Autodesk Inventor part; units mm, degrees
ref_plane "YZ Plane" through (0, 0, 0) normal (1, 0, 0) x (0, 1, 0)
ref_plane "XZ Plane" through (0, 0, 0) normal (0, 1, 0) x (-1, 0, 0)
ref_plane "XY Plane" through (0, 0, 0) normal (0, 0, 1) x (1, 0, 0)
sketch "Sketch1" plane through (0, 0, 0) normal (0, 1, 0) x (-1, 0, 0)
  circle A0 centre (0, 0) radius 8.5
  line L0 (10, -11.1988) -> (10, 11.1988)
  line L1 (-10, 11.1988) -> (-10, -11.1988)
  line L2 (-10, -14.792) -> (10, 14.792) construction
  line L3 (10, -14.792) -> (-10, 14.792) construction
  line L4 (10, 11.1988) -> (-10, 11.1988) construction
  arc A1 (10, 11.1988) -> (-10, 11.1988) centre (0, -0.9197) ccw
  line L5 (14.8819, 0) -> (-15.6848, 0) construction
  arc A2 (-10, -11.1988) -> (10, -11.1988) centre (0, 0.9197) ccw
  circle A3 centre (0, 0) radius 9.5
  dimension "d0" = 17
  dimension "d1" = 20
  dimension "d2" = 1
extrude "Extrusion1" add sketch "Sketch1" along normal blind 75 contours A3
extrude "Extrusion2" add sketch "Sketch1" along normal blind 3
sketch "Sketch2" plane through (0, 0, 0) normal (0, 0, 1) x (1, 0, 0)
  line L0 (9.5, 75) -> (-9.5, 75)
  line L1 (-9.5, 75) -> (-7.5, 75)
  line L2 (-7.5, 75) -> (-3.4008, 77.3135)
  line L3 (-3.4008, 77.3135) -> (-2.4311, 78.5256)
  line L4 (-2.4311, 78.5256) -> (-1.9463, 85.879)
  line L5 (-1.9463, 85.879) -> (-0.9463, 85.879)
  line L6 (-0.9463, 85.879) -> (-0.9463, 78.5256)
  line L7 (-0.9463, 78.5256) -> (-3.4008, 75)
  line L8 (-3.4008, 75) -> (-9.5, 75)
  line L9 (-3.4008, 77.3135) -> (-9.5, 75)
  line L10 (0, -17.1758) -> (0, 103.0548)
  point P0 (0, 0)
  dimension "d7" = 2
  dimension "d8" = 1
revolve "Revolution1" add sketch "Sketch2" angle 360 about axis through (0, -10, 0) along (0, 1, 0)
properties part number "Small Syringe"
For this review, take the finished solid that the model builds, in its own axes (mm). A direction names the side the tool comes from. Give positions to 0.01 mm unless a question says otherwise; leave off trailing zeros. Loops run counter-clockwise (first coordinate to the right, second up) from the corner with the lowest first, then second, coordinate; pieces in that order, holes last.
Item 1: Insertion check: pin 1 (12 mm diameter, centred on y = 18.5, z = -1, fed in from -X); pin 2 (4 mm diameter, centred on x = -4.5, y = 26.5, fed in from -Z); pin 3 (10 mm diameter, centred on x = -1, z = 10, fed in from +Y). Each pin has a flat end and moves straight along its axis. Give the tip position at first contact, or say it passes through.
Item 2: Draft analysis for pull direction Y (two halves, no side actions). For faces 1 (the conical face through (-2.09, 82.15, -0.66)), 2 (the cylindrical face through (-4.57, 38.496, -7.167)), 3 (the cylindrical face through (-4.38, 38.5, 8.43)), state which applies: +Y half, -Y half, draft (parallel to the pull), parting line (faces both ways), or undercut.
Item 3: Take a section at B-B, the plane x = 0. State the section outline as (y, z) points.
Item 4: For line 1 along Z through (x, y) = (0, 36); line 2 along Y through (x, z) = (3.75, 11.5); line 3 along Y through (x, z) = (3.75, 1.5), list the stretches that pass through material, from the lowest coordinate up.
Item 5: Take a section at C-C, the plane y = 71.5. State the section outline as (x, z) points, and give its area (3 significant figures).
Item 6: Tool access review of faces 4 (the cylindrical face through (0.205, 82.151, 0.924)), 5 (the flat face through (0, 3, 0)), 6 (the flat face through (10, 1, 0)): name each direction out of +Z, -Z, +X, -X, +Y, -Y from which nothing blocks a thin tool from reaching the whole face with its end or side.
Item 7: Take a section at A-A, the plane z = 0. State the section outline as (x, y) points.
Calculated:
1. pin 1: stops at x = -9.5
1. pin 2: stops at z = -9.17
1. pin 3: stops at y = 76.69
2. face 1: +Y half
2. face 2: undercut
2. face 3: draft
3. outline: (0, -14.79) - (3, -14.79) - (3, -9.5) - (75, -9.5) - (77.31, -3.4) - (78.53, -2.43) - (85.88, -1.95) - (85.88, -0.95) - (78.53, -0.95) - (75, -3.4) - (75, -8.5) - (3, -8.5) - (3, 8.5) - (75, 8.5) - (75, 3.4) - (78.53, 0.95) - (85.88, 0.95) - (85.88, 1.95) - (78.53, 2.43) - (77.31, 3.4) - (75, 9.5) - (3, 9.5) - (3, 14.79) - (0, 14.79) - close
4. line 1: z = -9.5 to -8.5, 8.5 to 9.5
4. line 2: y = 0 to 3
4. line 3: y = 0 to 3, 75 to 77.07
5. outline: circle Ø19 at (0, 0); hole circle Ø17 at (0, 0)
5. area: 56.5 mm2
6. face 4: +Y
6. face 5: none
6. face 6: +Z, -Z, +X, +Y, -Y
7. outline: (-10, 0) - (10, 0) - (10, 3) - (9.5, 3) - (9.5, 75) - (3.4, 77.31) - (2.43, 78.53) - (1.95, 85.88) - (0.95, 85.88) - (0.95, 78.53) - (3.4, 75) - (8.5, 75) - (8.5, 3) - (-8.5, 3) - (-8.5, 75) - (-3.4, 75) - (-0.95, 78.53) - (-0.95, 85.88) - (-1.95, 85.88) - (-2.43, 78.53) - (-3.4, 77.31) - (-9.5, 75) - (-9.5, 3) - (-10, 3) - close
